Model file for the job. Use its own axes, mm. Give positions to 0.01 mm unless a question says otherwise; leave off trailing zeros. Write each loop counter-clockwise with the first axis right and the second up, starting at its lowest first coordinate (ties: lowest second). Pieces come first, ordered by that corner, then holes.
```python
from build123d import *

# Parameters (mm, degrees)
F0_R     = 38.1
F1_DEPTH = 114.3
F2_T     = -2.54


# Not quite as in the source:
# - a fillet or chamfer that OpenCascade refuses, or shapes differently, is made with other operations: its cross-section is extruded or revolved along the edge and cut away or added


with BuildPart() as f1:
    # F0 (on Top) → F1 (new body)
    with BuildSketch(Plane.XY):
        Circle(F0_R)
    extrude(amount=F1_DEPTH)

    # F2
    f2_openings = [f1.faces().sort_by_distance(p)[0] for p in [
        (0, 0, 114.3),
    ]]
    offset(amount=F2_T, openings=f2_openings)

    # F3: fillet of radius 5.08 on 1 edges, made by hand

    # F3_s1 → F3_t2 (revolve, cut)
    with BuildSketch(Plane.XZ):
        with BuildLine():
            ThreePointArc((38.1, 109.9005909488), (37.4194090512, 112.4405909488), (35.56, 114.3))
            Line((35.56, 114.3), (38.1, 114.3))
            Line((38.1, 114.3), (38.1, 109.9005909488))
        make_face()
    revolve(axis=Axis((0, 0, 114.3), (0, 0, 1)), mode=Mode.SUBTRACT)


solid = f1.part
```
1. Pin check, flat tips, straight feed: P1, Ø1, axis at y = 6, z = 25.5, coming from the -X side; P2, Ø1.5, axis at x = 14, z = 42.5, coming from the +Y side; P3, Ø12, axis at y = -19, z = 45.5, coming from the +X side. Stop position of each tip, or through.
Calculated:
P1: stops at x = -37.7
P2: stops at y = 35.72
P3: stops at x = 35.81
2. Pull direction Y, two halves, no side cores. Call faces 1 (the cylindrical face through (-30.235, -23.183, 54.181)), 2 (the cylindrical face through (-7.709, -34.714, 57.638)), 3 (the flat face through (-1, 1, 0)): +Y half, -Y half, draft (parallel to the pull), parting line (faces both ways), or undercut.
Calculated:
face 1: parting line
face 2: undercut
face 3: draft
3. Slice it at B-B, the plane z = 33. Write the cut outline in (x, y).
Calculated:
outline: circle Ø76.2 at (0, 0); hole circle Ø71.12 at (0, 0)
4. Probe probe 1 along Y at (x, z) = (0, 91); probe 2 along X at (y, z) = (9.5, 74.5); probe 3 along Z at (x, y) = (16.5, -24). List the from-to ranges inside material, lowest first.
Calculated:
probe 1: y = -38.1 to -35.56, 35.56 to 38.1
probe 2: x = -36.9 to -34.27, 34.27 to 36.9
probe 3: z = 0 to 2.54
5. Slice it at A-A, the plane x = 0. Write the cut outline in (y, z).
Calculated:
outline: (-38.1, 0) - (38.1, 0) - (38.1, 109.9) arc R5.08 ccw to (35.56, 114.3) - (35.56, 2.54) - (-35.56, 2.54) - (-35.56, 114.3) arc R5.08 ccw to (-38.1, 109.9) - close
